Geometry check sheet. Reference: the model listing, model coordinates, mm. A direction names the side the tool comes from. Give positions to 0.01 mm unless a question says otherwise; leave off trailing zeros. Order: outer loops, then holes, each group sorted by start corner. A loop starts at its lowest first (then second) coordinate and runs counter-clockwise, first axis right, second up.
from build123d import *

# Parameters (mm, degrees)
BOSS_EXTRUDE1_DEPTH = 8
SKETCH2_R           = 1.25
BOSS_EXTRUDE2_DEPTH = 6
CUT_EXTRUDE1_START  = -8
SKETCH2_2_R         = 1.25
CUT_EXTRUDE1_DEPTH  = 6


with BuildPart() as part:
    # Sketch1 → Boss-Extrude1 (new body)
    with BuildSketch(Plane(origin=(0, 0, 0), x_dir=(1, 0, 0), z_dir=(0, 1, 0))):
        Polygon((0, 2.713546265), (-2.35, 1.356773133), (-2.35, -1.356773133), (0, -2.713546265), (2.35, -1.356773133), (2.35, 1.356773133), align=None)
    extrude(amount=BOSS_EXTRUDE1_DEPTH)

    # Sketch2 → Boss-Extrude2 (add)
    with BuildSketch(Plane(origin=(0, 8, 0), x_dir=(1, 0, 0), z_dir=(0, 1, 0))):
        Circle(SKETCH2_R)
    extrude(amount=BOSS_EXTRUDE2_DEPTH)

    # Sketch2<2> → Cut-Extrude1 (cut)
    with BuildSketch(Plane(origin=(0, 8, 0), x_dir=(1, 0, 0), z_dir=(0, 1, 0)).offset(CUT_EXTRUDE1_START)):
        Circle(SKETCH2_2_R)
    extrude(amount=CUT_EXTRUDE1_DEPTH, mode=Mode.SUBTRACT)


solid = part.part
Item 1: Sectioned sample at A-A (y = 3). Enter the section's corners in (x, z).
Reported:
outline: (-2.35, -1.36) - (0, -2.71) - (2.35, -1.36) - (2.35, 1.36) - (0, 2.71) - (-2.35, 1.36) - close; hole circle Ø2.5 at (0, 0)
Item 2: Draft check along X on faces 1 (the cylindrical face through (-0.27, 2.96, 1.22)), 2 (the flat face through (-2.35, 4, 0)), 3 (the cylindrical face through (-0.27, 10.96, 1.22)). Enter one of: released by +X, released by -X, zero draft, split by the parting line, or undercut.
Reported:
face 1: undercut
face 2: released by -X
face 3: split by the parting line
Item 3: Sectioned sample at C-C (x = -1.1). Enter the section's corners in (y, z).
Reported:
outline: (0, -2.08) - (8, -2.08) - (8, -0.59) - (14, -0.59) - (14, 0.59) - (8, 0.59) - (8, 2.08) - (0, 2.08) - (0, 0.59) - (6, 0.59) - (6, -0.59) - (0, -0.59) - close
Item 4: Sectioned sample at B-B (y = 7.5). Enter the section's corners in (x, z), and give its area (3 significant figures).
Reported:
outline: (-2.35, -1.36) - (0, -2.71) - (2.35, -1.36) - (2.35, 1.36) - (0, 2.71) - (-2.35, 1.36) - close
area: 19.1 mm2
Item 5: Scan lines: L1, parallel to X at y = 1.75, z = 0; L2, parallel to Y at x = 1.75, z = 0.05; L3, parallel to X at y = 11, z = -0.4. Record each from-to range of solid material in increasing order.
Reported:
L1: x = -2.35 to -1.25, 1.25 to 2.35
L2: y = 0 to 8
L3: x = -1.18 to 1.18
Item 6: Set-up check for faces 4 (the flat face through (0, 6, 0)), 5 (the flat face through (-1, 8, 1)), 6 (the flat face through (1.191, 3.944, -2.026)): record each of +Z, -Z, +X, -X, +Y, -Y from which the full face is reachable in a straight line by a thin tool's end or side.
Reported:
face 4: -Y
face 5: +Y
face 6: -Z, +X, +Y, -Y
Item 7: Gauge pin test, flat end, axial feed: pin 1 (1.5 mm diameter, centred on x = 0.5, y = 4.5, fed in from +Z). Record the tip position at first contact, or that the pin passes through.
Reported:
pin 1: stops at z = 2.71
Item 8: Sectioned sample at D-D (z = 0.85). Enter the section's corners in (x, y).
Reported:
outline: (-2.35, 0) - (-0.92, 0) - (-0.92, 6) - (0.92, 6) - (0.92, 0) - (2.35, 0) - (2.35, 8) - (0.92, 8) - (0.92, 14) - (-0.92, 14) - (-0.92, 8) - (-2.35, 8) - close
